from build123d import *

# Parameters (mm, degrees)
EXTRUDE_1_DEPTH     = 0.5
SKETCH_3_W          = 25
SKETCH_3_H          = 35
CUT_EXTRUDE_1_DEPTH = 114.058613257
SKETCH_4_W          = 10
SKETCH_4_H          = 35
CUT_EXTRUDE_2_DEPTH = 114.058613257
SKETCH_5_W          = 50
SKETCH_5_H          = 20
CUT_EXTRUDE_3_DEPTH = 114.058613257
SKETCH_6_W          = 10
SKETCH_6_H          = 20
CUT_EXTRUDE_4_DEPTH = 114.058613257
EXTRUDE_2_DEPTH     = 0.5
CUT_EXTRUDE_5_DEPTH = 119.289418767
FILLET_1_R          = 5
FILLET_2_R          = 20


with BuildPart() as part:
    # ｽｹｯﾁ1 → ﾎﾞｽ - 押し出し1 (new, symmetric)
    with BuildSketch(Plane(origin=(0, 0, 0), x_dir=(1, 0, 0), z_dir=(0, 1, 0))):
        with BuildLine():
            Line((62.68888804, 92.5), (-62.68888804, 92.5))
            add(Edge.make_bspline(
                [(-62.68888804, 92.5), (-67.396314277, 0), (-62.68888804, -92.5)],
                knots=[4.444925752, 4.444925752, 4.444925752, 4.979852209, 4.979852209, 4.979852209], degree=2, weights=[1, 0.964444431, 1]))
            Line((-62.68888804, -92.5), (62.68888804, -92.5))
            add(Edge.make_bspline(
                [(62.68888804, -92.5), (67.396314277, 0), (62.68888804, 92.5)],
                knots=[1.303333099, 1.303333099, 1.303333099, 1.838259555, 1.838259555, 1.838259555], degree=2, weights=[1, 0.964444431, 1]))
        make_face()
    extrude(amount=EXTRUDE_1_DEPTH, both=True)

    # ｽｹｯﾁ3 → ｶｯﾄ - 押し出し1 (cut, through all)
    with BuildSketch(Plane(origin=(0, 0.5, 0), x_dir=(1, 0, 0), z_dir=(0, 1, 0))):
        with Locations((-52.5, 75)):
            Rectangle(SKETCH_3_W, SKETCH_3_H)
    extrude(amount=-CUT_EXTRUDE_1_DEPTH, mode=Mode.SUBTRACT)

    # ｽｹｯﾁ4 → ｶｯﾄ - 押し出し2 (cut, through all)
    with BuildSketch(Plane(origin=(0, 0.5, 0), x_dir=(1, 0, 0), z_dir=(0, 1, 0))):
        with Locations((60, 75)):
            Rectangle(SKETCH_4_W, SKETCH_4_H)
    extrude(amount=-CUT_EXTRUDE_2_DEPTH, mode=Mode.SUBTRACT)

    # ｽｹｯﾁ5 → ｶｯﾄ - 押し出し3 (cut, through all)
    with BuildSketch(Plane(origin=(0, 0.5, 0), x_dir=(1, 0, 0), z_dir=(0, 1, 0))):
        with Locations((-40, -82.5)):
            Rectangle(SKETCH_5_W, SKETCH_5_H)
    extrude(amount=-CUT_EXTRUDE_3_DEPTH, mode=Mode.SUBTRACT)

    # ｽｹｯﾁ6 → ｶｯﾄ - 押し出し4 (cut, through all)
    with BuildSketch(Plane(origin=(0, 0.5, 0), x_dir=(1, 0, 0), z_dir=(0, 1, 0))):
        with Locations((60, -82.5)):
            Rectangle(SKETCH_6_W, SKETCH_6_H)
    extrude(amount=-CUT_EXTRUDE_4_DEPTH, mode=Mode.SUBTRACT)

    # ｽｹｯﾁ7 → ﾎﾞｽ - 押し出し2 (add, symmetric)
    with BuildSketch(Plane(origin=(0, 0, 0), x_dir=(1, 0, 0), z_dir=(0, 1, 0))):
        with BuildLine():
            Line((-15, -92.5), (55, -92.5))
            ThreePointArc((55, -92.5), (20, -98.825030024), (-15, -92.5))
        make_face()
    extrude(amount=EXTRUDE_2_DEPTH, both=True)

    # ｽｹｯﾁ8 → ｶｯﾄ - 押し出し5 (cut, through all)
    with BuildSketch(Plane(origin=(0, 0.5, 0), x_dir=(1, 0, 0), z_dir=(0, 1, 0))):
        with BuildLine():
            ThreePointArc((-40, 67.5), (-32.677669545, 85.177669514), (-15.000000044, 92.5))
            Line((-15.000000044, 92.5), (-40, 92.5))
            Line((-40, 92.5), (-40, 67.5))
        make_face()
        with BuildLine():
            Line((55, 67.5), (55, 92.5))
            Line((55, 92.5), (30, 92.5))
            ThreePointArc((30, 92.5), (47.67766953, 85.17766953), (55, 67.5))
        make_face()
    extrude(amount=-CUT_EXTRUDE_5_DEPTH, mode=Mode.SUBTRACT)

    # ﾌｨﾚｯﾄ1
    fillet_1_edges = [part.edges().sort_by_distance(p)[0] for p in [
        (-63.590195865, -0.25, 72.5),
        (63.590195865, -0.2499997, 72.5),
        (64.116831739, -0.25, -57.5),
    ]]
    fillet(fillet_1_edges, radius=FILLET_1_R)

    # ﾌｨﾚｯﾄ2
    fillet_2_edges = [part.edges().sort_by_distance(p)[0] for p in [
        (-15, 0, 92.5),
        (55, 0, 92.5),
    ]]
    fillet(fillet_2_edges, radius=FILLET_2_R)


solid = part.part
Read the model definition and answer for the solid it produces. Units are mm, in the model's axes. Coordinates: 2 decimals unless noted, no trailing zeros. Loops run counter-clockwise (first coordinate to the right, second up) from the corner with the lowest first, then second, coordinate; pieces in that order, holes last.
Q1. Each of these flat-tipped pins is pushed along its axis until it touches: pin 1 Ø0.5 at (x, y) = (57, 0) entering from +Z; pin 2 Ø0.5 at (y, z) = (0, -61.5) entering from -X; pin 3 Ø0.5 at (y, z) = (0, 75) entering from +X. Where does it stop, or does it pass through?
Q2. The part is cut by section A-A on x = -46.5. Write down the section's boundary in (y, z), and give its area (3 significant figures).
Q3. The part is cut by section B-B on x = -4.5. Write down the section's boundary in (y, z).
Q4. Consider probe 1 along Z at (x, y) = (21.5, 0); probe 2 along X at (y, z) = (-0.05, -65.5); probe 3 along X at (y, z) = (0.45, -1). Determine where each line is inside the solid, lowest interval first.
Results below:
1. pin 1: stops at z = 72.5
1. pin 2: stops at x = -40
1. pin 3: stops at x = 55
2. outline: (-0.5, -57.5) - (0.5, -57.5) - (0.5, 72.5) - (-0.5, 72.5) - close
2. area: 130 mm2
3. outline: (-0.5, -92.5) - (0.5, -92.5) - (0.5, 95.01) - (-0.5, 95.01) - close
4. probe 1: z = -92.5 to 98.81
4. probe 2: x = -40 to 55
4. probe 3: x = -65 to 65
